Autodesk Inventor part; units mm, degrees
ref_plane "YZ Plane" through (0, 0, 0) normal (1, 0, 0) x (0, 1, 0)
ref_plane "XZ Plane" through (0, 0, 0) normal (0, 1, 0) x (-1, 0, 0)
ref_plane "XY Plane" through (0, 0, 0) normal (0, 0, 1) x (1, 0, 0)
sketch "Sketch1" plane through (0, 0, 0) normal (0, 0, 1) x (1, 0, 0)
  line L0 (25, -2.55) -> (-25, -2.55)
  line L1 (-25, -2.55) -> (-25, 2.55)
  line L2 (-25, 2.55) -> (25, 2.55)
  line L3 (25, 2.55) -> (25, -2.55)
  line L4 (25, -2.55) -> (-25, 2.55) construction
  line L5 (-25, -2.55) -> (25, 2.55) construction
  point P0 (0, 0)
  dimension "d0" = 50
  dimension "d1" = 5.1
extrude "Extrusion1" add sketch "Sketch1" along normal blind 45.1
sketch "Sketch2" plane through (-25, -2.55, 0) normal (0, -1, 0) x (1, 0, 0)
  line L0 (50, 0) -> (0, 0)
  line L1 (10, 0) -> (20.05, 0)
  line L2 (20.05, 0) -> (20.05, 5.1)
  line L3 (20.05, 5.1) -> (10, 5.1)
  line L4 (10, 5.1) -> (10, 0)
  line L5 (40.05, 0) -> (30, 0)
  line L6 (30, 0) -> (30, 5.1)
  line L7 (30, 5.1) -> (40.05, 5.1)
  line L8 (40.05, 5.1) -> (40.05, 0)
  line L9 (50, 0) -> (50, 45.1)
  line L10 (0, 0) -> (0, 45.1)
  point P0 (25, 0)
  point P1 (40.05, 2.55)
  point P2 (10, 2.55)
  dimension "d5" = 5.1
  dimension "d9" = 5.1
  dimension "d17" = 9.95
  dimension "d24" = 9.95
  dimension "d25" = 10.05
  dimension "d26" = 10.05
extrude "Extrusion2" cut sketch "Sketch2" against normal blind 45.1
sketch "Sketch3" plane through (-25, -2.55, 45.1) normal (0, -1, 0) x (1, 0, 0)
  circle A0 centre (25, -5.6) radius 3.45
  line L0 (0, 0) -> (50, 0)
  circle A1 centre (25, -5.6) radius 12.05
  line L1 (50, 0) -> (0, 0)
  line L2 (0, 0) -> (0, 10.45)
  line L3 (0, 10.45) -> (50, 10.45)
  line L4 (50, 10.45) -> (50, 0)
  line L5 (0, -45.1) -> (0, 0)
  line L6 (50, -45.1) -> (50, 0)
  line L7 (0, -44.9) -> (50, -44.9)
  line L8 (50, -44.9) -> (50, -45.1)
  line L9 (50, -45.1) -> (0, -45.1)
  line L10 (0, -45.1) -> (0, -44.9)
  point P0 (25, -45.1)
  point P1 (14.3303, 0)
  point P2 (35.6697, 0)
  dimension "d12" = 6.9
  dimension "d13" = 5.6
  dimension "d14" = 25
  dimension "d19" = 24.1
  dimension "d20" = 16.05
  dimension "d27" = 0.2
extrude "Extrusion3" cut sketch "Sketch3" against normal blind 45.1 contours A0 | L0 A1 picked at (25.1386, -0.7251)
extrude "Extrusion4" add sketch "Sketch3" against normal up to surface (5.1 mm away) contours L2 L3 L4 L0 A1
extrude "Extrusion5" cut sketch "Sketch3" against normal through all contours L7 L6 L9 L5
fillet "Fillet1" radius 15 2 edges at (25, 0, 55.55) (-25, 0, 55.55)
equation "\"d24\" = d23"
equation "\"d26\" = d25"
equation "\"d23\" = d17"
properties part number "motorholder1A" material "Polycarbonate, Smoke"
The model under review builds one solid part; all positions refer to its coordinate system, in mm. A direction names the side the tool comes from. Round coordinates to 2 decimals unless told otherwise and drop trailing zeros. Order: outer loops, then holes, each group sorted by start corner. A loop starts at its lowest first (then second) coordinate and runs counter-clockwise, first axis right, second up. Notation, with made-up numbers: M -21,-20 L -5,-20 A30 cw -5,6 Z; hole C 2.25,-22 d11. An arc over 180 degrees is marked long. Use a Markdown table: item, result.
1) Consider section C-C (y = -0.8). Write out the cut boundary in (x, z), then the cut area to 3 significant figures.
Report:
| item | result |
|---|---|
| outline | M -25,0.2 L -15,0.2 L -15,5.1 L -4.95,5.1 L -4.95,0.2 L 5,0.2 L 5,5.1 L 15.05,5.1 L 15.05,0.2 L 25,0.2 L 25,40.55 A15 ccw 10,55.55 L -10,55.55 A15 ccw -25,40.55 Z; hole C 0,39.5 d24.1 |
| area | 2,120 mm^2 |
2) Tool access review of faces 1 (the face through (20, 0, 0.2)), 2 (the face through (10, 0, 5.1)): name each direction out of +Z, -Z, +X, -X, +Y, -Y from which nothing blocks a thin tool from reaching the whole face with its end or side.
Report:
| item | result |
|---|---|
| face 1 | -Z, +X, -X, +Y, -Y |
| face 2 | -Z, +Y, -Y |
3) Draft analysis for pull direction X (two halves, no side actions). For faces 3 (the face through (0, 0, 0.2)), 4 (the face through (20.49, 0.04, 51.27)), 5 (the face through (-10, 0, 5.1)), state which applies: released by +X, released by -X, zero draft, split by the parting line, or undercut.
Report:
| item | result |
|---|---|
| face 3 | zero draft |
| face 4 | released by +X |
| face 5 | undercut |
4) Wall thickness on line 1 along X through (y, z) = (-0.3, 39.5); line 2 along Z through (x, y) = (0, 0.85); line 3 along Z through (x, y) = (-11, 1.75): over which ranges is each line inside the solid? List them lowest first. Write a range as [from, to].
Report:
| item | result |
|---|---|
| line 1 | [-25, -12.05], [12.05, 25] |
| line 2 | [0.2, 27.45], [51.55, 55.55] |
| line 3 | [5.1, 34.58], [44.42, 55.52] |
5) Consider section D-D (x = -20). Write out the cut boundary in (y, z), then the cut area to 3 significant figures.
Report:
| item | result |
|---|---|
| outline | M -2.55,0.2 L 2.55,0.2 L 2.55,51.73 L -2.55,51.73 Z |
| area | 263 mm^2 |
6) Insertion check: pin 1 (1.5 mm diameter, centred on x = 12.5, y = -0.5, fed in from -Z); pin 2 (1 mm diameter, centred on y = 1.5, z = 42, fed in from +X). Each pin has a flat end and moves straight along its axis. Give the tip position at first contact, or say it passes through.
Report:
| item | result |
|---|---|
| pin 1 | z = 5.1 |
| pin 2 | x = 24.97 |
7) Consider section A-A (z = 39.5). Write out the cut boundary in (x, y).
Report:
| item | result |
|---|---|
| outline | M -25,-2.55 L -12.05,-2.55 L -12.05,2.55 L -25,2.55 Z; M 12.05,-2.55 L 25,-2.55 L 25,2.55 L 12.05,2.55 Z |
8) Consider section B-B (x = 0). Write out the cut boundary in (y, z).
Report:
| item | result |
|---|---|
| outline | M -2.55,0.2 L 2.55,0.2 L 2.55,27.45 L -2.55,27.45 Z; M -2.55,51.55 L 2.55,51.55 L 2.55,55.55 L -2.55,55.55 Z |
